Autodesk Inventor part; units mm, degrees
ref_plane "YZ Plane" through (0, 0, 0) normal (1, 0, 0) x (0, 1, 0)
ref_plane "XZ Plane" through (0, 0, 0) normal (0, 1, 0) x (-1, 0, 0)
ref_plane "XY Plane" through (0, 0, 0) normal (0, 0, 1) x (1, 0, 0)
sketch "Sketch1" plane through (0, 0, 0) normal (0, 1, 0) x (-1, 0, 0)
  circle A0 centre (0, 0) radius 304.8
  dimension "d0" = 609.6
extrude "Extrusion1" add sketch "Sketch1" along normal blind 3.175
sketch "Sketch2" plane through (0, 3.175, 0) normal (0, 1, 0) x (1, 0, 0)
  circle A0 centre (0, 0) radius 304.8
  circle A1 centre (0, 0) radius 6.35
  dimension "d3" = 12.7
extrude "Extrusion2" cut sketch "Sketch2" against normal blind 3.175 contours A1
sketch "Sketch3" plane through (0, 3.175, 0) normal (0, 1, 0) x (1, 0, 0)
  circle A0 centre (0, 0) radius 6.35
  circle A1 centre (0, 292.1) radius 4.6302
  dimension "d6" = 292.1
hole "Hole1" at (0, 3.175, -292.1) direction (0, -1, 0) diameter 4.4958 end through all countersink diameter 8.4328 countersink angle 82
pattern_circular "Circular Pattern1" count 4 over 360 about axis through (0, 3.175, 0) along (0, -1, 0) of "Hole1"
sketch "Sketch9" plane through (0, 3.175, 0) normal (0, 1, 0) x (1, 0, 0)
  circle A0 centre (0, 0) radius 304.8
  line L0 (0, 0) -> (14.7527, -55.0578) construction
  line L1 (0, 0) -> (57, 0) construction
  line L2 (0, 0) -> (-55.0578, 14.7527) construction
  line L3 (0, 0) -> (57, 0) construction
  circle A1 centre (42.4264, 42.4264) radius 7.377
  circle A2 centre (14.7527, -55.0578) radius 7.6366
  circle A3 centre (-55.0578, 14.7527) radius 7.2502
  circle A4 centre (0, 0) radius 6.35
  line L4 (0, 0) -> (42.4264, 42.4264) construction
  line L5 (0, 0) -> (60, 0) construction
  dimension "d85" = 57
  dimension "d86" = 75
  dimension "d87" = 57
  dimension "d88" = 195
  dimension "d96" = 60
  dimension "d97" = 45
hole "Hole7" at (-55.0578, 3.175, -14.7527) at (42.4264, 3.175, -42.4264) at (14.7527, 3.175, 55.0578) direction (0, -1, 0) diameter 6.6 end through all
properties part number "2f1bd" material "Aluminum 6061"
Verification items for the finished model (mm, model axes). Coordinates: 2 decimals unless noted, no trailing zeros. Write each loop counter-clockwise with the first axis right and the second up, starting at its lowest first coordinate (ties: lowest second). Pieces come first, ordered by that corner, then holes. Notation, with made-up numbers: M -15,1.25 L 37,1.25 A16 ccw 37,27.25 Z; hole C 49.5,29 d2. An arc over 180 degrees is marked long. Use a Markdown table: item, result.
Q1. Sectioned sample at B-B, the plane z = -183.5. Record the boundary of the cut face in (x, y) (3 decimals).
Reply:
| item | result |
|---|---|
| outline | M -243.374,0 L 243.374,0 L 243.374,3.175 L -243.374,3.175 Z |
Q2. Thickness scan on line 1 (Z direction, x = 0, y = 2.4); line 2 (Z direction, x = 215.5, y = 1.25); line 3 (Z direction, x = 41, y = 1.9). Record the ranges inside material, lowest first.
Reply:
| item | result |
|---|---|
| line 1 | z = -304.8 to -295.64, -288.56 to -6.35, 6.35 to 288.56, 295.64 to 304.8 |
| line 2 | z = -215.55 to 215.55 |
| line 3 | z = -302.03 to -45.4, -39.45 to 302.03 |
Q3. Go/stop test with flat-tipped pins: P1, Ø2.5, axis at x = 0, z = 292.1, coming from the -Y side; P2, Ø7, axis at x = -292.1, z = 0, coming from the +Y side; P3, Ø1, axis at x = 234.5, y = 1.5, coming from the -Z side. Record where each tip stops, or that it passes through.
Reply:
| item | result |
|---|---|
| P1 | passes through |
| P2 | stops at y = 2.35 |
| P3 | stops at z = -195.31 |
Q4. Sectioned sample at A-A, the plane x = -163.5. Record the boundary of the cut face in (y, z) (3 decimals), plus the area to 3 significant figures.
Reply:
| item | result |
|---|---|
| outline | M 0,-257.237 L 3.175,-257.237 L 3.175,257.237 L 0,257.237 Z |
| area | 1,630 mm² |
